```python
from build123d import *

# Parameters (mm, degrees)
SKETCH1_W           = 10
SKETCH1_H           = 100
BOSS_EXTRUDE1_DEPTH = 5
SKETCH2_W           = 10
SKETCH2_H           = 100
BOSS_EXTRUDE2_DEPTH = 5
SKETCH3_W           = 20
SKETCH3_H           = 5
BOSS_EXTRUDE3_DEPTH = 20
FILLET1_R           = 10
CUT_EXTRUDE1_REACH  = 60.523
SKETCH4_R           = 2.15
FILLET2_R           = 10


with BuildPart() as part:
    # Sketch1 → Boss-Extrude1 (new body)
    with BuildSketch(Plane(origin=(0, 0, 0), x_dir=(1, 0, 0), z_dir=(0, 1, 0))):
        with Locations((-5, 0)):
            Rectangle(SKETCH1_W, SKETCH1_H)
    extrude(amount=BOSS_EXTRUDE1_DEPTH)

    # Sketch2 → Boss-Extrude2 (add)
    with BuildSketch(Plane(origin=(0, 5, 0), x_dir=(1, 0, 0), z_dir=(0, 1, 0))):
        with Locations((-5, 0)):
            Rectangle(SKETCH2_W, SKETCH2_H)
    extrude(amount=BOSS_EXTRUDE2_DEPTH)

    # Sketch3 → Boss-Extrude3 (add)
    with BuildSketch(Plane.ZY.offset(10)):
        with Locations((0, 2.5)):
            Rectangle(SKETCH3_W, SKETCH3_H)
    extrude(amount=BOSS_EXTRUDE3_DEPTH)

    # Fillet1
    fillet1_edges = [part.edges().sort_by_distance(p)[0] for p in [
        (-30, 2.5, 10),
        (-30, 2.5, -10),
    ]]
    fillet(fillet1_edges, radius=FILLET1_R - 0.0001)  # a hair under: the kernel refuses the full size

    # Sketch4 → Cut-Extrude1 (cut, up to next)
    with BuildSketch(Plane(origin=(0, 5, 0), x_dir=(1, 0, 0), z_dir=(0, 1, 0)), mode=Mode.PRIVATE) as cut_extrude1_sk1:
        with Locations(Location((-20, 0, 0), (0, 0, 270))):
            Circle(SKETCH4_R)
    cut_extrude1_tool1 = extrude(cut_extrude1_sk1.sketch, amount=-CUT_EXTRUDE1_REACH, mode=Mode.PRIVATE) & part.part
    add(cut_extrude1_tool1.solids().sort_by_distance((-20, 5, 0))[0], mode=Mode.SUBTRACT)

    # Fillet2
    fillet2_edges = [part.edges().sort_by_distance(p)[0] for p in [
        (-10, 5, -50),
        (-10, 5, 50),
    ]]
    fillet(fillet2_edges, radius=FILLET2_R - 0.0001)  # a hair under: the kernel refuses the full size


solid = part.part
```
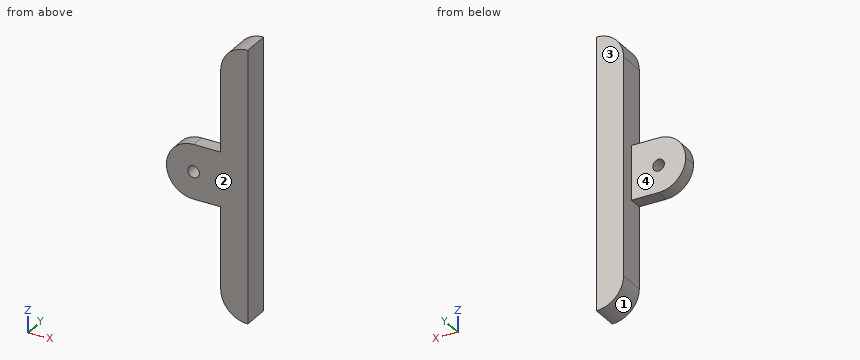
Geometry check sheet. Reference: the model listing, model coordinates, mm. Face numbers are marked on the shaded views. A direction names the side the tool comes from. Give positions to 0.01 mm unless a question says otherwise; leave off trailing zeros. Order: outer loops, then holes, each group sorted by start corner. A loop starts at its lowest first (then second) coordinate and runs counter-clockwise, first axis right, second up. Notation, with made-up numbers: (54.25, 9.5) - (82.25, 9.5) arc R15 cw to (82.25, 26.5) - close; hole circle Ø3 at (86.25, 57). An arc over 180 degrees is marked (long way). Write item = value, one per line. Start each with the question number.
1) Section check D-D (x = -17). Enter the section's corners in (y, z), then the cut area to 3 significant figures.
2) Draft check along X on the marked faces 1 and 2. Enter one of: released by +X, released by -X, zero draft, split by the parting line, or undercut.
3) Scan lines: L1, parallel to X at y = 1.85, z = 0; L2, parallel to Z at x = -13, y = 3.5; L3, parallel to Y at x = -15, z = 9. Record each from-to range of solid material in increasing order.
4) Access from +Z, -Z, +X, -X, +Y, -Y to the whole of each face (thin tool, end or side, straight path). Record for the marked faces 3 and 4.
5) Gauge pin test, flat ends, axial feed: pin 1 Ø5.5 at (x, y) = (-15, 3.5) entering from +Z; pin 2 Ø5 at (y, z) = (6, 31.5) entering from +X; pin 3 Ø6 at (y, z) = (6.5, -22) entering from -X; pin 4 Ø5.5 at (x, y) = (-13, 3.5) entering from -Z. Record the tip position at first contact, or that the pin passes through.
6) Section check B-B (z = 20). Enter the section's corners in (x, y), then the cut area to 3 significant figures.
Geometry check:
q1.outline = (0, -10) - (5, -10) - (5, 10) - (0, 10) - close
q1.area = 100 mm2
q2.face_1 = released by -X
q2.face_2 = zero draft
q3.L1 = -30 to -22.15, -17.85 to 0
q3.L2 = -10 to 10
q3.L3 = 0 to 5
q4.face_3 = +Z, -Z, +X, -X, +Y
q4.face_4 = +Z, -Z, -X, +Y
q5.pin_1 = 10
q5.pin_2 = 0
q5.pin_3 = -10
q5.pin_4 = -10
q6.outline = (-10, 0) - (0, 0) - (0, 10) - (-10, 10) - close
q6.area = 100 mm2
